Check sheet for the modelled part. Datum: model origin and axes. Units: mm. A direction names the side the tool comes from. Give positions to 0.01 mm unless a question says otherwise; leave off trailing zeros. Order: outer loops, then holes, each group sorted by start corner. A loop starts at its lowest first (then second) coordinate and runs counter-clockwise, first axis right, second up. Notation, with made-up numbers: (74.5, 7) - (85.5, 7) arc R27 cw to (85.5, 34) - close; hole circle Ø6 at (87, 66.25). An arc over 180 degrees is marked (long way). Answer in a Markdown table with one row per item.
from build123d import *

# Parameters (mm, degrees)
CROQUIS1_W              = 52.5
CROQUIS1_H              = 42
CROQUIS1_W_2            = 45.5
CROQUIS1_H_2            = 35
SALIENTE_EXTRUIR1_DEPTH = 10
CROQUIS3_W              = 52.5
CROQUIS3_H              = 42
SALIENTE_EXTRUIR2_DEPTH = 3
CROQUIS4_W              = 38
CROQUIS4_H              = 3
SALIENTE_EXTRUIR3_DEPTH = 8
CROQUIS5_R              = 2
CORTAR_EXTRUIR1_DEPTH   = 1
CROQUIS6_R              = 1.6
CORTAR_EXTRUIR2_DEPTH   = 4
CROQUIS7_W              = 3
CROQUIS7_H              = 25
SALIENTE_EXTRUIR4_DEPTH = 8
CROQUIS8_R              = 2
CORTAR_EXTRUIR3_DEPTH   = 1
CROQUIS9_R              = 1.6
CORTAR_EXTRUIR4_DEPTH   = 3
CHAFL_N1_SIZE           = 1
REDONDEO2_R             = 1


with BuildPart() as part:
    # Croquis1 → Saliente-Extruir1 (new body)
    with BuildSketch(Plane.XY):
        Rectangle(CROQUIS1_W, CROQUIS1_H)
        Rectangle(CROQUIS1_W_2, CROQUIS1_H_2, mode=Mode.SUBTRACT)
    extrude(amount=SALIENTE_EXTRUIR1_DEPTH)

    # Croquis3 → Saliente-Extruir2 (add)
    with BuildSketch(Plane.XY):
        Rectangle(CROQUIS3_W, CROQUIS3_H)
    extrude(amount=-SALIENTE_EXTRUIR2_DEPTH)

    # Croquis4 → Saliente-Extruir3 (add)
    with BuildSketch(Plane.XZ.offset(21)):
        with Locations((0, -1.5)):
            Rectangle(CROQUIS4_W, CROQUIS4_H)
    extrude(amount=SALIENTE_EXTRUIR3_DEPTH)

    # Croquis5 → Cortar-Extruir1 (cut)
    with BuildSketch(Plane.XY):
        with Locations((-12, -25)):
            Circle(CROQUIS5_R)
        with Locations((-6, -25)):
            Circle(CROQUIS5_R)
        with Locations((0, -25)):
            Circle(CROQUIS5_R)
        with Locations((6, -25)):
            Circle(CROQUIS5_R)
        with Locations((12, -25)):
            Circle(CROQUIS5_R)
    extrude(amount=-CORTAR_EXTRUIR1_DEPTH, mode=Mode.SUBTRACT)

    # Croquis6 → Cortar-Extruir2 (cut)
    with BuildSketch(Plane.XY.offset(-1)):
        with Locations((-12, -25)):
            Circle(CROQUIS6_R)
        with Locations((-6, -25)):
            Circle(CROQUIS6_R)
        with Locations((0, -25)):
            Circle(CROQUIS6_R)
        with Locations((6, -25)):
            Circle(CROQUIS6_R)
        with Locations((12, -25)):
            Circle(CROQUIS6_R)
    extrude(amount=-CORTAR_EXTRUIR2_DEPTH, mode=Mode.SUBTRACT)

    # Croquis7 → Saliente-Extruir4 (add)
    with BuildSketch(Plane(origin=(26.25, 0, 0), x_dir=(0, 0, -1), z_dir=(1, 0, 0))):
        with Locations((1.5, 0)):
            Rectangle(CROQUIS7_W, CROQUIS7_H)
    extrude(amount=SALIENTE_EXTRUIR4_DEPTH)

    # Croquis8 → Cortar-Extruir3 (cut)
    with BuildSketch(Plane.XY):
        with Locations((30.25, 6)):
            Circle(CROQUIS8_R)
        with Locations((30.25, 0)):
            Circle(CROQUIS8_R)
        with Locations((30.25, -6)):
            Circle(CROQUIS8_R)
    extrude(amount=-CORTAR_EXTRUIR3_DEPTH, mode=Mode.SUBTRACT)

    # Croquis9 → Cortar-Extruir4 (cut)
    with BuildSketch(Plane(origin=(0, 0, -3), x_dir=(-1, 0, 0), z_dir=(0, 0, -1))):
        with Locations((-30.25, 6)):
            Circle(CROQUIS9_R)
        with Locations((-30.25, 0)):
            Circle(CROQUIS9_R)
        with Locations((-30.25, -6)):
            Circle(CROQUIS9_R)
    extrude(amount=-CORTAR_EXTRUIR4_DEPTH, mode=Mode.SUBTRACT)

    # Chaflán1
    chafl_n1_edges = [part.edges().sort_by_distance(p)[0] for p in [
        (26.25, -21, 3.5),
        (-26.25, -21, 3.5),
        (-26.25, 21, 3.5),
        (26.25, 21, 3.5),
    ]]
    chamfer(chafl_n1_edges, length=CHAFL_N1_SIZE)

    # Redondeo2
    redondeo2_edges = [part.edges().sort_by_distance(p)[0] for p in [
        (34.25, 12.5, -1.5),
        (34.25, -12.5, -1.5),
        (19, -29, -1.5),
        (-19, -29, -1.5),
    ]]
    fillet(redondeo2_edges, radius=REDONDEO2_R)


solid = part.part
(1) Mould release check, pull along X, two halves, no side actions. Record for faces 3 (the flat face through (19, -24, -2)), 4 (the flat face through (30, 12.5, -1)), 5 (the flat face through (-22.75, 0, 5)): pulls with the +X half, pulls with the -X half, needs draft (parallel to the pull), parting line crosses it, or undercut.
Geometry says:
| item | result |
|---|---|
| face 3 | pulls with the +X half |
| face 4 | needs draft |
| face 5 | undercut |
(2) Access from +Z, -Z, +X, -X, +Y, -Y to the whole of each face (thin tool, end or side, straight path). Record for faces 1 (the cylindrical face through (32.097, -6.766, -0.493)), 2 (the cylindrical face through (31.85, 0.07, -2.01)).
Geometry says:
| item | result |
|---|---|
| face 1 | +Z |
| face 2 | +Z, -Z |
(3) Cross-section at C-C, the plane x = 30.25. Record the cut outline in (y, z).
Geometry says:
| item | result |
|---|---|
| outline | (-12.5, -3) - (-7.6, -3) - (-7.6, -1) - (-8, -1) - (-8, 0) - (-12.5, 0) - close; (-4.4, -3) - (-1.6, -3) - (-1.6, -1) - (-2, -1) - (-2, 0) - (-4, 0) - (-4, -1) - (-4.4, -1) - close; (1.6, -3) - (4.4, -3) - (4.4, -1) - (4, -1) - (4, 0) - (2, 0) - (2, -1) - (1.6, -1) - close; (7.6, -3) - (12.5, -3) - (12.5, 0) - (8, 0) - (8, -1) - (7.6, -1) - close |
(4) Thickness scan on L1, parallel to Y at x = 30.25, z = -1.7; L2, parallel to Y at x = 30.25, z = -0.25; L3, parallel to Y at x = -9.5, z = 0.75. Record the ranges inside material, lowest first.
Geometry says:
| item | result |
|---|---|
| L1 | -12.5 to -7.6, -4.4 to -1.6, 1.6 to 4.4, 7.6 to 12.5 |
| L2 | -12.5 to -8, -4 to -2, 2 to 4, 8 to 12.5 |
| L3 | -21 to -17.5, 17.5 to 21 |
(5) Cross-section at A-A, the plane x = 12. Record the cut outline in (y, z), then the cut area to 3 significant figures.
Geometry says:
| item | result |
|---|---|
| outline | (-29, -3) - (-26.6, -3) - (-26.6, -1) - (-27, -1) - (-27, 0) - (-29, 0) - close; (-23.4, -3) - (21, -3) - (21, 10) - (17.5, 10) - (17.5, 0) - (-17.5, 0) - (-17.5, 10) - (-21, 10) - (-21, 0) - (-23, 0) - (-23, -1) - (-23.4, -1) - close |
| area | 210 mm² |
(6) Cross-section at B-B, the plane y = 0. Record the cut outline in (x, z), then the cut area to 3 significant figures.
Geometry says:
| item | result |
|---|---|
| outline | (-26.25, -3) - (28.65, -3) - (28.65, -1) - (28.25, -1) - (28.25, 0) - (26.25, 0) - (26.25, 10) - (22.75, 10) - (22.75, 0) - (-22.75, 0) - (-22.75, 10) - (-26.25, 10) - close; (31.85, -3) - (34.25, -3) - (34.25, 0) - (32.25, 0) - (32.25, -1) - (31.85, -1) - close |
| area | 241 mm² |
(7) Cross-section at D-D, the plane z = 4.5. Record the cut outline in (x, y).
Geometry says:
| item | result |
|---|---|
| outline | (-26.25, -20) - (-25.25, -21) - (25.25, -21) - (26.25, -20) - (26.25, 20) - (25.25, 21) - (-25.25, 21) - (-26.25, 20) - close; hole (-22.75, -17.5) - (22.75, -17.5) - (22.75, 17.5) - (-22.75, 17.5) - close |
(8) Gauge pin test, flat ends, axial feed: P1, Ø5, axis at x = 6, y = -25, coming from the +Z side; P2, Ø1.5, axis at x = 10.5, z = 7, coming from the -Y side; P3, Ø2.5, axis at y = -23, z = -1.5, coming from the -X side. Record the tip position at first contact, or that the pin passes through.
Geometry says:
| item | result |
|---|---|
| P1 | z = 0 |
| P2 | y = -21 |
| P3 | x = -19 |
